Geometry: final body of the model. Coordinates: model frame, mm. A direction names the side the tool comes from. Round coordinates to 2 decimals unless told otherwise and drop trailing zeros. Write each loop counter-clockwise with the first axis right and the second up, starting at its lowest first coordinate (ties: lowest second). Pieces come first, ordered by that corner, then holes. Notation, with made-up numbers: (-8.75, -34) -> (44.25, -34) arc R12 ccw to (44.25, -13) -> close; hole circle Ø5 at (84.5, 77.25). An arc over 180 degrees is marked (long way). One line per item, written item: value. Start each with the question number.
from build123d import *

# Parameters (mm, degrees)
SKETCH1_W           = 55
SKETCH1_H           = 44
BOSS_EXTRUDE1_DEPTH = 1.55
SKETCH2_W           = 14.5
SKETCH2_H           = 14.3
BOSS_EXTRUDE2_DEPTH = 7.1
SKETCH3_W           = 13.85
SKETCH3_H           = 6.5
SKETCH3_W_2         = 12.45
SKETCH3_H_2         = 1.497681088
CUT_EXTRUDE1_DEPTH  = 13.3
SKETCH4_W           = 8.95
SKETCH4_H           = 7.5
BOSS_EXTRUDE3_DEPTH = 2.85
CUT_EXTRUDE2_DEPTH  = 7.5
SKETCH5_3_W         = 7.15
SKETCH5_3_H         = 0.2
CUT_EXTRUDE3_DEPTH  = 7
BOSS_EXTRUDE4_DEPTH = 1.5


with BuildPart() as part:
    # Sketch1 → Boss-Extrude1 (new body)
    with BuildSketch(Plane(origin=(0, 0, 0), x_dir=(0, 1, 0), z_dir=(0, 0, 1))):
        Rectangle(SKETCH1_W, SKETCH1_H)
    extrude(amount=BOSS_EXTRUDE1_DEPTH)

    # Sketch2 → Boss-Extrude2 (add)
    with BuildSketch(Plane.XY.offset(1.55)):
        with Locations((13.1, -21.35)):
            Rectangle(SKETCH2_W, SKETCH2_H)
    extrude(amount=BOSS_EXTRUDE2_DEPTH)

    # Sketch3 → Cut-Extrude1 (cut)
    with BuildSketch(Plane.XZ.offset(28.5)):
        with Locations((13.1, 5.1)):
            Rectangle(SKETCH3_W, SKETCH3_H)
        with Locations((13.1, 6.101159456)):
            Rectangle(SKETCH3_W_2, SKETCH3_H_2, mode=Mode.SUBTRACT)
    extrude(amount=-CUT_EXTRUDE1_DEPTH, mode=Mode.SUBTRACT)

    # Sketch4 → Boss-Extrude3 (add)
    with BuildSketch(Plane.XY.offset(1.55)):
        with Locations((-13.025, 23.75)):
            Rectangle(SKETCH4_W, SKETCH4_H)
    extrude(amount=BOSS_EXTRUDE3_DEPTH)

    # Sketch5 → Cut-Extrude2 (cut)
    with BuildSketch(Plane(origin=(0, 27.5, 0), x_dir=(-1, 0, 0), z_dir=(0, 1, 0))):
        with BuildLine():
            Line((8.55, 4.4), (8.55, 2.975))
            ThreePointArc((8.55, 2.975), (8.910359128, 3.926260685), (9.810540583, 4.4))
            Line((9.810540583, 4.4), (8.55, 4.4))
        make_face()
        with BuildLine():
            Line((8.55, 1.55), (9.810540583, 1.55))
            ThreePointArc((9.810540583, 1.55), (8.910359128, 2.023739315), (8.55, 2.975))
            Line((8.55, 2.975), (8.55, 1.55))
        make_face()
        with BuildLine():
            Line((17.5, 1.55), (17.5, 2.975))
            ThreePointArc((17.5, 2.975), (17.139640872, 2.023739315), (16.239459417, 1.55))
            Line((16.239459417, 1.55), (17.5, 1.55))
        make_face()
        with BuildLine():
            Line((17.5, 4.4), (16.239459417, 4.4))
            ThreePointArc((16.239459417, 4.4), (17.139640872, 3.926260685), (17.5, 2.975))
            Line((17.5, 2.975), (17.5, 4.4))
        make_face()
    extrude(amount=-CUT_EXTRUDE2_DEPTH, mode=Mode.SUBTRACT)

    # Sketch5<3> → Cut-Extrude3 (cut)
    with BuildSketch(Plane(origin=(0, 27.5, 0), x_dir=(-1, 0, 0), z_dir=(0, 1, 0))):
        with BuildLine():
            Line((9.95, 1.719461162), (16.1, 1.719461162))
            ThreePointArc((16.1, 1.719461162), (17.355538838, 2.975), (16.1, 4.230538838))
            Line((16.1, 4.230538838), (9.95, 4.230538838))
            ThreePointArc((9.95, 4.230538838), (8.694461162, 2.975), (9.95, 1.719461162))
        make_face()
        with Locations((13.025, 2.975)):
            Rectangle(SKETCH5_3_W, SKETCH5_3_H, mode=Mode.SUBTRACT)
    extrude(amount=-CUT_EXTRUDE3_DEPTH, mode=Mode.SUBTRACT)

    # Sketch6 → Boss-Extrude4 (add)
    with BuildSketch(Plane.XY.offset(1.55)):
        Polygon((19.35, 23.5), (18.85, 22.633974596), (10.35, 22.633974596), (9.85, 23.5), (8.85, 23.5), (8.85, 12.3), (20.35, 12.3), (20.35, 23.5), align=None)
    extrude(amount=BOSS_EXTRUDE4_DEPTH)


solid = part.part
(1) Pull-direction query (Y, two-part tool) for faces 5 (the face through (13, -14.2, 5)), 6 (the face through (0, 0, 1.55)), 7 (the face through (-13, 24, 1.719)), 8 (the face through (15, 22.634, 2)); classes: pulls with the +Y half, pulls with the -Y half, needs draft (parallel to the pull), parting line crosses it, or undercut.
(2) Section query D-D (x = 3.5). Output: boundary loops of the cut face in (y, z).
(3) Section query A-A (y = -23.5). Output: boundary loops of the cut face in (x, z) (3 decimals).
(4) Set-up query: faces 1 (the face through (13, -22, 6.85)), 2 (the face through (15, 12.3, 2)), 3 (the face through (20.35, -21, 5)), 4 (the face through (-13, 24, 3.075)). Return all of +Z, -Z, +X, -X, +Y, -Y with unobstructed straight access to the full face (end or side cutting, diameter ignored); none if empty.
(5) Line query: probe 1 along X at (y, z) = (-23, 5.75) (3 decimals); probe 2 along Z at (x, y) = (15, -22.5); probe 3 along Z at (x, y) = (-13, 21.5) (3 decimals). Output: solid intervals per line, ascending.
(6) Pin query (flat end, axial travel): pin 1 (0.5 mm diameter, centred on x = -7, z = 0.5, fed in from -Y); pin 2 (1.6 mm diameter, centred on x = 13.5, z = 2.5, fed in from +Y); pin 3 (12 mm diameter, centred on x = 5, y = 16, fed in from +Z); pin 4 (5 mm diameter, centred on x = -12, z = 7.5, fed in from -Y). Return the tip coordinate at first contact, or that it passes through.
(7) Section query B-B (y = 13). Output: boundary loops of the cut face in (x, z).
(8) Section query C-C (z = 7.5). Output: boundary loops of the cut face in (x, y) (3 decimals).
Results list:
1. face 5: undercut
1. face 6: undercut
1. face 7: needs draft
1. face 8: pulls with the +Y half
2. outline: (-27.5, 0) -> (27.5, 0) -> (27.5, 1.55) -> (-27.5, 1.55) -> close
3. outline: (-22, 0) -> (22, 0) -> (22, 1.55) -> (20.35, 1.55) -> (20.35, 8.65) -> (5.85, 8.65) -> (5.85, 1.55) -> (-22, 1.55) -> close; (6.875, 5.352) -> (19.325, 5.352) -> (19.325, 6.85) -> (6.875, 6.85) -> close; hole (6.175, 1.85) -> (20.025, 1.85) -> (20.025, 8.35) -> (6.175, 8.35) -> close
4. face 1: -Y
4. face 2: +Z, +X, -X
4. face 3: +Z, +X, +Y, -Y
4. face 4: +Y
5. probe 1: x = 5.85 to 6.175, 6.875 to 19.325, 20.025 to 20.35
5. probe 2: z = 0 to 1.85, 5.35 to 6.85, 8.35 to 8.65
5. probe 3: z = 0 to 1.719, 2.875 to 3.075, 4.231 to 4.4
6. pin 1: stops at y = -27.5
6. pin 2: stops at y = 22.63
6. pin 3: stops at z = 3.05
6. pin 4: passes through
7. outline: (-22, 0) -> (22, 0) -> (22, 1.55) -> (20.35, 1.55) -> (20.35, 3.05) -> (8.85, 3.05) -> (8.85, 1.55) -> (-22, 1.55) -> close
8. outline: (5.85, -28.5) -> (6.175, -28.5) -> (6.175, -15.2) -> (20.025, -15.2) -> (20.025, -28.5) -> (20.35, -28.5) -> (20.35, -14.2) -> (5.85, -14.2) -> close
